Can you work these out from the model? Positions are in its coordinate system, mm. Round coordinates to 2 decimals unless told otherwise and drop trailing zeros. Write each loop counter-clockwise with the first axis right and the second up, starting at its lowest first coordinate (ties: lowest second). Pieces come first, ordered by that corner, then holes. Notation, with made-up numbers: (80, 32.5) -> (124, 32.5) arc R23 ccw to (124, 58.5) -> close; hole circle Ø7 at (84, 88.5). An arc over 180 degrees is marked (long way). Use CSV: the item, a comma, the result in double quotes.
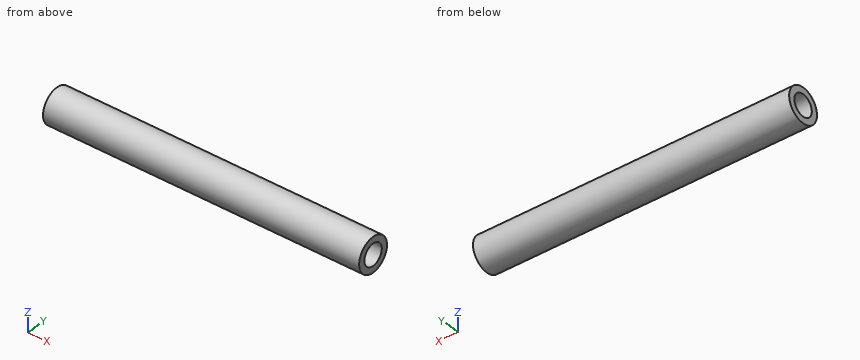
```python
from build123d import *

# Parameters (mm, degrees)
SKETCH1_R           = 4
BOSS_EXTRUDE1_DEPTH = 37
SKETCH2_R           = 2.5
CUT_EXTRUDE1_DEPTH  = 15


with BuildPart() as part:
    # Sketch1 → Boss-Extrude1 (new, symmetric)
    with BuildSketch(Plane(origin=(0, 0, 0), x_dir=(0, 0, -1), z_dir=(1, 0, 0))):
        Circle(SKETCH1_R)
    extrude(amount=BOSS_EXTRUDE1_DEPTH, both=True)

    # Sketch2 → Cut-Extrude1 (cut)
    with BuildSketch(Plane(origin=(37, 0, 0), x_dir=(0, 0, -1), z_dir=(1, 0, 0))):
        Circle(SKETCH2_R)
    cut_extrude1 = extrude(amount=-CUT_EXTRUDE1_DEPTH, mode=Mode.SUBTRACT)

    # Mirror1: Cut-Extrude1 across plane
    add(cut_extrude1.mirror(Plane(origin=(0, 0, 0), x_dir=(0, 0, 1), z_dir=(1, 0, 0))), mode=Mode.SUBTRACT)


solid = part.part
```
Q1. Suppose I cut it at A-A (z = 0). Write out the boundary of the cut face in (x, y).
Resolved:
outline,"(-37, -4) -> (37, -4) -> (37, -2.5) -> (22, -2.5) -> (22, 2.5) -> (37, 2.5) -> (37, 4) -> (-37, 4) -> (-37, 2.5) -> (-22, 2.5) -> (-22, -2.5) -> (-37, -2.5) -> close"
Q2. Will these pins go through, and if not, where does the flat tip stop? P1, Ø2, axis at x = 14.5, z = 2.5, coming from the -Y side; P2, Ø2, axis at y = 2, z = -0.5, coming from the +X side; P3, Ø4, axis at y = 0, z = 0, coming from the +X side; P4, Ø1, axis at y = -1.5, z = 0.5, coming from the -X side.
Resolved:
P1,"stops at y = -3.71"
P2,"stops at x = 37"
P3,"stops at x = 22"
P4,"stops at x = -22"
Q3. Suppose I cut it at C-C (x = 14). Write out the boundary of the cut face in (y, z), and give its area (3 significant figures).
Resolved:
outline,"circle Ø8 at (0, 0)"
area,"50.3 mm^2"
Q4. Please list where these lines run through material, in increasing order: probe 1 along Y at (x, z) = (34.25, 0); probe 2 along X at (y, z) = (-0.25, -1.75); probe 3 along Y at (x, z) = (23, 0.5).
Resolved:
probe 1,"y = -4 to -2.5, 2.5 to 4"
probe 2,"x = -22 to 22"
probe 3,"y = -3.97 to -2.45, 2.45 to 3.97"
